```python
from build123d import *

# Parameters (mm, degrees)
SKETCH1_W           = 120
SKETCH1_H           = 120
BOSS_EXTRUDE1_DEPTH = 15
CUT_EXTRUDE4_REACH  = 17
SKETCH7_R           = 2.5
SKETCH7_R_2         = 3


with BuildPart() as part:
    # Sketch1 → Boss-Extrude1 (new body)
    with BuildSketch(Plane.XY):
        Rectangle(SKETCH1_W, SKETCH1_H)
    extrude(amount=-BOSS_EXTRUDE1_DEPTH)

    # Sketch7 → Cut-Extrude4 (cut, up to next)
    with BuildSketch(Plane(origin=(0, 0, -15), x_dir=(-1, 0, 0), z_dir=(0, 0, -1)), mode=Mode.PRIVATE) as cut_extrude4_sk1:
        with Locations((-36, -40)):
            Circle(SKETCH7_R)
    cut_extrude4_tool1 = extrude(cut_extrude4_sk1.sketch, amount=-CUT_EXTRUDE4_REACH, mode=Mode.PRIVATE) & part.part
    add(cut_extrude4_tool1.solids().sort_by_distance((36, -40, -15))[0], mode=Mode.SUBTRACT)
    # Sketch7 → Cut-Extrude4 (cut, up to next)
    with BuildSketch(Plane(origin=(0, 0, -15), x_dir=(-1, 0, 0), z_dir=(0, 0, -1)), mode=Mode.PRIVATE) as cut_extrude4_sk2:
        with Locations((-36, 40)):
            Circle(SKETCH7_R)
    cut_extrude4_tool2 = extrude(cut_extrude4_sk2.sketch, amount=-CUT_EXTRUDE4_REACH, mode=Mode.PRIVATE) & part.part
    add(cut_extrude4_tool2.solids().sort_by_distance((36, 40, -15))[0], mode=Mode.SUBTRACT)
    # Sketch7 → Cut-Extrude4 (cut, up to next)
    with BuildSketch(Plane(origin=(0, 0, -15), x_dir=(-1, 0, 0), z_dir=(0, 0, -1)), mode=Mode.PRIVATE) as cut_extrude4_sk3:
        with Locations((36, -40)):
            Circle(SKETCH7_R)
    cut_extrude4_tool3 = extrude(cut_extrude4_sk3.sketch, amount=-CUT_EXTRUDE4_REACH, mode=Mode.PRIVATE) & part.part
    add(cut_extrude4_tool3.solids().sort_by_distance((-36, -40, -15))[0], mode=Mode.SUBTRACT)
    # Sketch7 → Cut-Extrude4 (cut, up to next)
    with BuildSketch(Plane(origin=(0, 0, -15), x_dir=(-1, 0, 0), z_dir=(0, 0, -1)), mode=Mode.PRIVATE) as cut_extrude4_sk4:
        with Locations((36, 40)):
            Circle(SKETCH7_R)
    cut_extrude4_tool4 = extrude(cut_extrude4_sk4.sketch, amount=-CUT_EXTRUDE4_REACH, mode=Mode.PRIVATE) & part.part
    add(cut_extrude4_tool4.solids().sort_by_distance((-36, 40, -15))[0], mode=Mode.SUBTRACT)
    # Sketch7 → Cut-Extrude4 (cut, up to next)
    with BuildSketch(Plane(origin=(0, 0, -15), x_dir=(-1, 0, 0), z_dir=(0, 0, -1)), mode=Mode.PRIVATE) as cut_extrude4_sk5:
        with Locations((50, 0)):
            Circle(SKETCH7_R_2)
    cut_extrude4_tool5 = extrude(cut_extrude4_sk5.sketch, amount=-CUT_EXTRUDE4_REACH, mode=Mode.PRIVATE) & part.part
    add(cut_extrude4_tool5.solids().sort_by_distance((-50, 0, -15))[0], mode=Mode.SUBTRACT)
    # Sketch7 → Cut-Extrude4 (cut, up to next)
    with BuildSketch(Plane(origin=(0, 0, -15), x_dir=(-1, 0, 0), z_dir=(0, 0, -1)), mode=Mode.PRIVATE) as cut_extrude4_sk6:
        with Locations((-50, 0)):
            Circle(SKETCH7_R_2)
    cut_extrude4_tool6 = extrude(cut_extrude4_sk6.sketch, amount=-CUT_EXTRUDE4_REACH, mode=Mode.PRIVATE) & part.part
    add(cut_extrude4_tool6.solids().sort_by_distance((50, 0, -15))[0], mode=Mode.SUBTRACT)


solid = part.part
```
Verification items for the finished model (mm, model axes). Coordinates: 2 decimals unless noted, no trailing zeros. Write each loop counter-clockwise with the first axis right and the second up, starting at its lowest first coordinate (ties: lowest second). Pieces come first, ordered by that corner, then holes. Notation, with made-up numbers: M 11,61.5 L 22,61.5 A21 ccw 22,84.5 Z; hole C -10.5,23 d9. An arc over 180 degrees is marked long. One line per item, written item: value.
Item 1: Section check B-B, the plane x = -50. Record the boundary of the cut face in (y, z).
Check sheet entries:
outline: M -60,-15 L -3,-15 L -3,0 L -60,0 Z; M 3,-15 L 60,-15 L 60,0 L 3,0 Z
Item 2: Scan lines: line 1 along Y through (x, z) = (36, -7.5); line 2 along Y through (x, z) = (-50, -11.5). Record each from-to range of solid material in increasing order.
Check sheet entries:
line 1: y = -60 to -42.5, -37.5 to 37.5, 42.5 to 60
line 2: y = -60 to -3, 3 to 60
Item 3: Section check A-A, the plane y = 40. Record the boundary of the cut face in (x, z).
Check sheet entries:
outline: M -60,-15 L -38.5,-15 L -38.5,0 L -60,0 Z; M -33.5,-15 L 33.5,-15 L 33.5,0 L -33.5,0 Z; M 38.5,-15 L 60,-15 L 60,0 L 38.5,0 Z
Item 4: Gauge pin test, flat ends, axial feed: pin 1 Ø8 at (x, y) = (-22, -28) entering from +Z; pin 2 Ø3 at (x, y) = (-36, 40) entering from +Z. Record the tip position at first contact, or that the pin passes through.
Check sheet entries:
pin 1: stops at z = 0
pin 2: passes through
Item 5: Mould release check, pull along Y, two halves, no side actions. Record for faces 1 (the cylindrical face through (33.69, 39.04, -7.6)), 2 (the flat face through (-1, -60, -7)), 3 (the cylindrical face through (33.69, -40.96, -7.6)), 4 (the flat face through (-1, 1, -15)): pulls with the +Y half, pulls with the -Y half, needs draft (parallel to the pull), parting line crosses it, or undercut.
Check sheet entries:
face 1: undercut
face 2: pulls with the -Y half
face 3: undercut
face 4: needs draft
Item 6: Section check C-C, the plane x = 36. Record the boundary of the cut face in (y, z).
Check sheet entries:
outline: M -60,-15 L -42.5,-15 L -42.5,0 L -60,0 Z; M -37.5,-15 L 37.5,-15 L 37.5,0 L -37.5,0 Z; M 42.5,-15 L 60,-15 L 60,0 L 42.5,0 Z
